```python
from build123d import *

# Parameters (mm, degrees)
SKETCH1_R           = 4.7625
SKETCH1_R_2         = 45.72
BOSS_EXTRUDE1_DEPTH = 6.35


with BuildPart() as part:
    # Sketch1 → Boss-Extrude1 (new body)
    with BuildSketch(Plane.XY):
        with BuildLine():
            Line((-215.322727273, 31.220796272), (-12.7, 68.685751798))
            ThreePointArc((-12.7, 68.685751798), (69.85, 0), (-12.7, -68.685751798))
            Line((-12.7, -68.685751798), (-215.322727273, -31.220796272))
            ThreePointArc((-215.322727273, -31.220796272), (-225.746283623, -27.308293553), (-234.178235051, -20.037777778))
            ThreePointArc((-234.178235051, -20.037777778), (-234.582694183, -16.670432885), (-231.715411546, -14.859))
            Line((-231.715411546, -14.859), (-187.265411546, -14.859))
            ThreePointArc((-187.265411546, -14.859), (-172.406411546, 0), (-187.265411546, 14.859))
            Line((-187.265411546, 14.859), (-231.715411546, 14.859))
            ThreePointArc((-231.715411546, 14.859), (-234.582694183, 16.670432885), (-234.178235051, 20.037777778))
            ThreePointArc((-234.178235051, 20.037777778), (-225.746283623, 27.308293553), (-215.322727273, 31.220796272))
        make_face()
        with Locations((0, 57.15)):
            Circle(SKETCH1_R, mode=Mode.SUBTRACT)
        with Locations((49.493351826, 28.575)):
            Circle(SKETCH1_R, mode=Mode.SUBTRACT)
        with Locations((49.493351826, -28.575)):
            Circle(SKETCH1_R, mode=Mode.SUBTRACT)
        with Locations((0, -57.15)):
            Circle(SKETCH1_R, mode=Mode.SUBTRACT)
        with Locations((-49.493351826, -28.575)):
            Circle(SKETCH1_R, mode=Mode.SUBTRACT)
        with Locations((-49.493351826, 28.575)):
            Circle(SKETCH1_R, mode=Mode.SUBTRACT)
        Circle(SKETCH1_R_2, mode=Mode.SUBTRACT)
    extrude(amount=BOSS_EXTRUDE1_DEPTH)


solid = part.part
```
Could you check a few things on this model? Use its own coordinates, in mm. A direction names the side the tool comes from. Round coordinates to 2 decimals unless told otherwise and drop trailing zeros. Order: outer loops, then holes, each group sorted by start corner. A loop starts at its lowest first (then second) coordinate and runs counter-clockwise, first axis right, second up. Notation, with made-up numbers: (59.25, -38) -> (103.25, -38) arc R33 ccw to (103.25, -2) -> close; hole circle Ø4 at (-14, 37.5). An arc over 180 degrees is marked (long way). One line per question, with ' | ' between items.
Q1. We'd pull the mould along X, two halves only. Please class faces 3 (the face through (-80, 1, 0)), 4 (the face through (-225.88, 27.23, 3.13)), 5 (the face through (54.036, -27.144, 3.131)): released by +X, released by -X, zero draft, split by the parting line, or undercut.
Computed values:
face 3: zero draft | face 4: released by -X | face 5: undercut
Q2. I'm going to push flat-ended pins straight in: pin 1 (1.9 mm diameter, centred on x = -209, z = 4, fed in from -Y); pin 2 (1 mm diameter, centred on y = -16.5, z = 3, fed in from +X); pin 3 (1 mm diameter, centred on x = -21, z = 3, fed in from +Y). Where does each tip first touch, or does it pass through?
Computed values:
pin 1: y = -32.57 | pin 2: x = 67.99 | pin 3: y = 67.24
Q3. If we section it at A-A on y = 0: Write out the boundary of the cut face in (x, z), plus the area to 3 significant figures.
Computed values:
outline: (-172.41, 0) -> (-45.72, 0) -> (-45.72, 6.35) -> (-172.41, 6.35) -> close; (45.72, 0) -> (69.85, 0) -> (69.85, 6.35) -> (45.72, 6.35) -> close | area: 958 mm²
Q4. If I drill on line 1 (Y direction, x = 0, z = 2); line 2 (X direction, y = -26, z = 5.25); line 3 (X direction, y = 29, z = 1.5), over which ranges is the centre line in solid material (lowest first)? Write a range as from..to.
Computed values:
line 1: -69.85..-61.91, -52.39..-45.72, 45.72..52.39, 61.91..69.85 | line 2: -227.77..-53.5, -45.49..-37.61, 37.61..45.49, 53.5..64.83 | line 3: -222.48..-54.24, -44.75..-35.35, 35.35..44.75, 54.24..63.55
Q5. If we section it at B-B on x = 0: Write out the boundary of the cut face in (y, z).
Computed values:
outline: (-69.85, 0) -> (-61.91, 0) -> (-61.91, 6.35) -> (-69.85, 6.35) -> close; (-52.39, 0) -> (-45.72, 0) -> (-45.72, 6.35) -> (-52.39, 6.35) -> close; (45.72, 0) -> (52.39, 0) -> (52.39, 6.35) -> (45.72, 6.35) -> close; (61.91, 0) -> (69.85, 0) -> (69.85, 6.35) -> (61.91, 6.35) -> close
Q6. If we section it at C-C on x = -50: Write out the boundary of the cut face in (y, z), plus the area to 3 significant figures.
Computed values:
outline: (-61.79, 0) -> (-33.31, 0) -> (-33.31, 6.35) -> (-61.79, 6.35) -> close; (-23.84, 0) -> (23.84, 0) -> (23.84, 6.35) -> (-23.84, 6.35) -> close; (33.31, 0) -> (61.79, 0) -> (61.79, 6.35) -> (33.31, 6.35) -> close | area: 664 mm²
Q7. Which directions (+Z, -Z, +X, -X, +Y, -Y) give clear straight access to the entire face, cutting with the end or side of a thin tool? Please do faces 1 (the face through (-209, 14.859, 3)), 2 (the face through (-1.03, -61.8, 3.13)).
Computed values:
face 1: +Z, -Z, -X | face 2: +Z, -Z
Q8. If we section it at D-D on z = 4.5: Give the number of separate pieces and of enclosed holes in the cut face, plus the area to 3 significant figures.
Computed values:
separate pieces: 1 | enclosed holes: 7 | area: 22,000 mm²
